Here's how the part is built. I have some questions about the finished solid (model axes, mm). Face numbers are marked on the shaded views. A direction names the side the tool comes from. Round coordinates to 2 decimals unless told otherwise and drop trailing zeros. Order: outer loops, then holes, each group sorted by start corner. A loop starts at its lowest first (then second) coordinate and runs counter-clockwise, first axis right, second up.
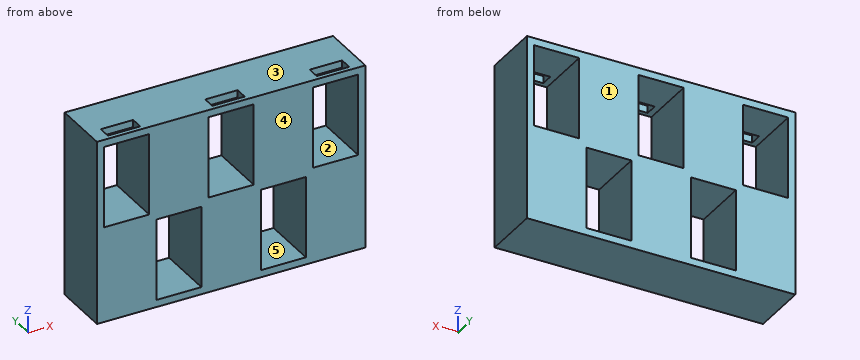
```python
from build123d import *

# Parameters (mm, degrees)
F0_W     = 74.4
F0_H     = 51.18
F0_W_2   = 12.48
F0_H_2   = 22.59
F1_DEPTH = 16
F2_W     = 9
F2_H     = 3.5
F3_DEPTH = 25


with BuildPart() as f1:
    # F0 (on Front) → F1 (new body)
    with BuildSketch(Plane.XZ):
        Rectangle(F0_W, F0_H)
        with Locations((-14.48, -12.295)):
            Rectangle(F0_W_2, F0_H_2, mode=Mode.SUBTRACT)
        with Locations((14.48, -12.295)):
            Rectangle(F0_W_2, F0_H_2, mode=Mode.SUBTRACT)
        with Locations((-28.96, 12.295)):
            Rectangle(F0_W_2, F0_H_2, mode=Mode.SUBTRACT)
        with Locations((0, 12.295)):
            Rectangle(F0_W_2, F0_H_2, mode=Mode.SUBTRACT)
        with Locations((28.96, 12.295)):
            Rectangle(F0_W_2, F0_H_2, mode=Mode.SUBTRACT)
    extrude(amount=F1_DEPTH)

    # F2 (on face) → F3 (cut)
    with BuildSketch(Plane(origin=(0, 0, 23.59), x_dir=(1, 0, 0), z_dir=(0, 0, -1))):
        with Locations((-0.005, 12.95)):
            Rectangle(F2_W, F2_H)
        with Locations((-28.955, 12.95)):
            Rectangle(F2_W, F2_H)
        with Locations((28.955, 12.95)):
            Rectangle(F2_W, F2_H)
    extrude(amount=-F3_DEPTH, mode=Mode.SUBTRACT)


solid = f1.part
```
1. If we section it at D-D, the plane x = -31.5: Write out the boundary of the cut face in (y, z), and give its area (3 significant figures).
Evaluation:
outline: (-16, -25.59) - (0, -25.59) - (0, 1) - (-16, 1) - close; (-16, 23.59) - (-14.7, 23.59) - (-14.7, 25.59) - (-16, 25.59) - close; (-11.2, 23.59) - (0, 23.59) - (0, 25.59) - (-11.2, 25.59) - close
area: 450 mm2
2. On a 3-axis mill with a long thin cutter (end or side, diameter ignored), from which of +Z, -Z, +X, -X, +Y, -Y can I reach the whole of each face in a straight line? I mean the marked faces 4 and 5. Say none if no direction works.
Evaluation:
face 4: +Z, -Z, +X, -X, -Y
face 5: +Y, -Y
3. If we section it at C-C, the plane y = -10: Write out the boundary of the cut face in (x, z), and give its area (3 significant figures).
Evaluation:
outline: (-37.2, -25.59) - (37.2, -25.59) - (37.2, 25.59) - (-37.2, 25.59) - close; hole (-35.2, 1) - (-22.72, 1) - (-22.72, 23.59) - (-35.2, 23.59) - close; hole (-20.72, -23.59) - (-8.24, -23.59) - (-8.24, -1) - (-20.72, -1) - close; hole (-6.24, 1) - (6.24, 1) - (6.24, 23.59) - (-6.24, 23.59) - close; hole (8.24, -23.59) - (20.72, -23.59) - (20.72, -1) - (8.24, -1) - close; hole (22.72, 1) - (35.2, 1) - (35.2, 23.59) - (22.72, 23.59) - close
area: 2,400 mm2
4. If we section it at A-A, the plane x = 11.5: Write out the boundary of the cut face in (y, z), and give its area (3 significant figures).
Evaluation:
outline: (-16, -25.59) - (0, -25.59) - (0, -23.59) - (-16, -23.59) - close; (-16, -1) - (0, -1) - (0, 25.59) - (-16, 25.59) - close
area: 457 mm2
5. I need wall thicknesses on probe 1 along X at (y, z) = (-12, -14); probe 2 along X at (y, z) = (-5.5, 13); probe 3 along Z at (x, y) = (23, -14). Which ranges of each line are inside material? Lowest first, please.
Evaluation:
probe 1: x = -37.2 to -20.72, -8.24 to 8.24, 20.72 to 37.2
probe 2: x = -37.2 to -35.2, -22.72 to -6.24, 6.24 to 22.72, 35.2 to 37.2
probe 3: z = -25.59 to 1, 23.59 to 25.59
6. If we mould it in two halves opening along Z, with no side actions, what happens to the marked faces 1, 2 and 3? For each: released by +Z, released by -Z, zero draft, split by the parting line, or undercut.
Evaluation:
face 1: zero draft
face 2: undercut
face 3: released by +Z
7. If we section it at B-B, the plane z = 12: Write out the boundary of the cut face in (x, y), and give its area (3 significant figures).
Evaluation:
outline: (-37.2, -16) - (-35.2, -16) - (-35.2, 0) - (-37.2, 0) - close; (-22.72, -16) - (-6.24, -16) - (-6.24, 0) - (-22.72, 0) - close; (6.24, -16) - (22.72, -16) - (22.72, 0) - (6.24, 0) - close; (35.2, -16) - (37.2, -16) - (37.2, 0) - (35.2, 0) - close
area: 591 mm2
